from build123d import *

# Parameters (mm, degrees)
F0_W     = 25.4
F0_H     = 25.4
F1_DEPTH = 6.35
F2_W     = 25.4
F2_H     = 15.24
F2_W_2   = 7.62
F3_DEPTH = 25.4
F4_R     = 7.62
F5_SIZE  = 20.32
F6_R     = 10.16
F7_R     = 3.302
F8_DEPTH = 20.321
F9_R     = 2


with BuildPart() as f1:
    # F0 (on Top) → F1 (new body)
    with BuildSketch(Plane.XY):
        Rectangle(F0_W, F0_H)
    extrude(amount=F1_DEPTH)

    # F2 (on face) → F3 (join)
    with BuildSketch(Plane.XY.offset(6.35)):
        Rectangle(F2_W, F2_H)
        with Locations((16.51, 0)):
            Rectangle(F2_W_2, F2_H)
    extrude(amount=F3_DEPTH)

    # F4
    f4_edges = [f1.edges().sort_by_distance(p)[0] for p in [
        (20.32, 0, 31.75),
    ]]
    fillet(f4_edges, radius=F4_R)

    # F5
    f5_edges = [f1.edges().sort_by_distance(p)[0] for p in [
        (-12.7, 0, 31.75),
    ]]
    chamfer(f5_edges, length=F5_SIZE)

    # F6
    f6_edges = [f1.edges().sort_by_distance(p)[0] for p in [
        (7.62, 0, 31.75),
    ]]
    fillet(f6_edges, radius=F6_R)

    # F7 (on face) → F8 (cut, through all)
    with BuildSketch(Plane.XZ.offset(7.62)):
        with Locations((12.7, 24.13)):
            Circle(F7_R)
    extrude(amount=-F8_DEPTH, mode=Mode.SUBTRACT)

    # F9
    f9_edges = [f1.edges().sort_by_distance(p)[0] for p in [
        (-4.027898, -7.62, 20.102102),
        (-4.027898, 7.62, 20.102102),
        (-12.7, 0, 11.43),
        (-12.7, -7.62, 8.89),
        (-12.7, 7.62, 8.89),
        (12.264205, -7.62, 31.75),
        (7.940346, -7.62, 30.976616),
        (18.088154, -7.62, 29.518154),
        (20.32, -7.62, 15.24),
        (12.264205, 7.62, 31.75),
        (7.940346, 7.62, 30.976616),
        (18.088154, 7.62, 29.518154),
        (20.32, 7.62, 15.24),
    ]]
    fillet(f9_edges, radius=F9_R)


solid = f1.part
For this review, take the finished solid that the model builds, in its own axes (mm). A direction names the side the tool comes from. Round coordinates to 2 decimals unless told otherwise and drop trailing zeros. Write each loop counter-clockwise with the first axis right and the second up, starting at its lowest first coordinate (ties: lowest second). Pieces come first, ordered by that corner, then holes. Notation, with made-up numbers: (72, 56) -> (90, 56) arc R22 cw to (90, 86) -> close; hole circle Ø10 at (78.5, 37.25). An arc over 180 degrees is marked (long way). Put each result on its own line as item: value.
Q1. Consider section D-D on y = 6.5. State the section outline as (x, z) points, and give its area (3 significant figures).
Determined:
outline: (-12.7, 0) -> (12.7, 0) -> (12.7, 6.35) -> (20.12, 6.35) -> (20.12, 24.13) arc R7.42 ccw to (12.7, 31.55) -> (11.83, 31.55) arc R9.96 ccw to (4.79, 28.63) -> (-11.97, 11.87) arc R1.8 ccw to (-12.5, 10.6) -> (-12.5, 6.35) -> (-12.7, 6.35) -> close; hole circle Ø6.6 at (12.7, 24.13)
area: 731 mm^2
Q2. The part is to be moulded in two halves that separate along Z. For faces 1 (the cylindrical face through (-3.45, 7.02, 19.87)), 2 (the flat face through (16, 0, 6.35)), 3 (the flat face through (12.7, 0, 3)), 4 (the cylindrical face through (12.27, -0.107, 27.404)), say which applies: released by +Z, released by -Z, zero draft, split by the parting line, or undercut.
Determined:
face 1: released by +Z
face 2: released by -Z
face 3: zero draft
face 4: undercut
Q3. Machinability: for faces 5 (the flat face through (7, -7.62, 15)), 6 (the flat face through (7, 7.62, 15)), 7 (the flat face through (20.32, 0, 15)), 8 (the flat face through (-3.85, -0.08, 20.28)), 9 (the cylindrical face through (-12.13, 7.02, 8.51)), which of the approach directions +Z, -Z, +X, -X, +Y, -Y give a long, thin tool a straight path to every point of the face, cutting with its end or side? Answer none if there is none.
Determined:
face 5: +Z, +X, -X, -Y
face 6: +Z, +X, -X, +Y
face 7: +Z, -Z, +X, +Y, -Y
face 8: +Z, -X, +Y, -Y
face 9: +Z, -X, +Y
Q4. Consider section A-A on y = -0.75. State the section outline as (x, z) points.
Determined:
outline: (-12.7, 0) -> (12.7, 0) -> (12.7, 6.35) -> (20.32, 6.35) -> (20.32, 24.13) arc R7.62 ccw to (12.7, 31.75) -> (11.83, 31.75) arc R10.16 ccw to (4.64, 28.77) -> (-12.11, 12.02) arc R2 ccw to (-12.7, 10.6) -> close; hole circle Ø6.6 at (12.7, 24.13)
Q5. Clearance check with flat-ended pins moving along their axes: pin 1 Ø8 at (y, z) = (-7.5, 18.5) entering from -X; pin 2 Ø2 at (x, y) = (-6.5, 6) entering from +Z; pin 3 Ø12 at (x, z) = (0.5, 25) entering from +Y; pin 4 Ø6 at (x, z) = (12.7, 24.13) entering from -Y. State where each tip first meets the part, or that it passes through.
Determined:
pin 1: stops at x = -9.29
pin 2: stops at z = 18.6
pin 3: stops at y = 7.62
pin 4: passes through
Q6. Consider section C-C on z = 3. State the section outline as (x, y) points.
Determined:
outline: (-12.7, -12.7) -> (12.7, -12.7) -> (12.7, 12.7) -> (-12.7, 12.7) -> close
Q7. Consider section B-B on y = 9.75. State the section outline as (x, z) points.
Determined:
outline: (-12.7, 0) -> (12.7, 0) -> (12.7, 6.35) -> (-12.7, 6.35) -> close
Q8. To check wall thickness, follow L1, parallel to Z at x = -1, y = 11.75; L2, parallel to X at y = -4, z = 4; L3, parallel to Y at x = 18.5, z = 24.5. State the ranges of each line that lie inside material, in increasing order. Write a range as [from, to].
Determined:
L1: z = [0, 6.35]
L2: x = [-12.7, 12.7]
L3: y = [-7.61, 7.61]
